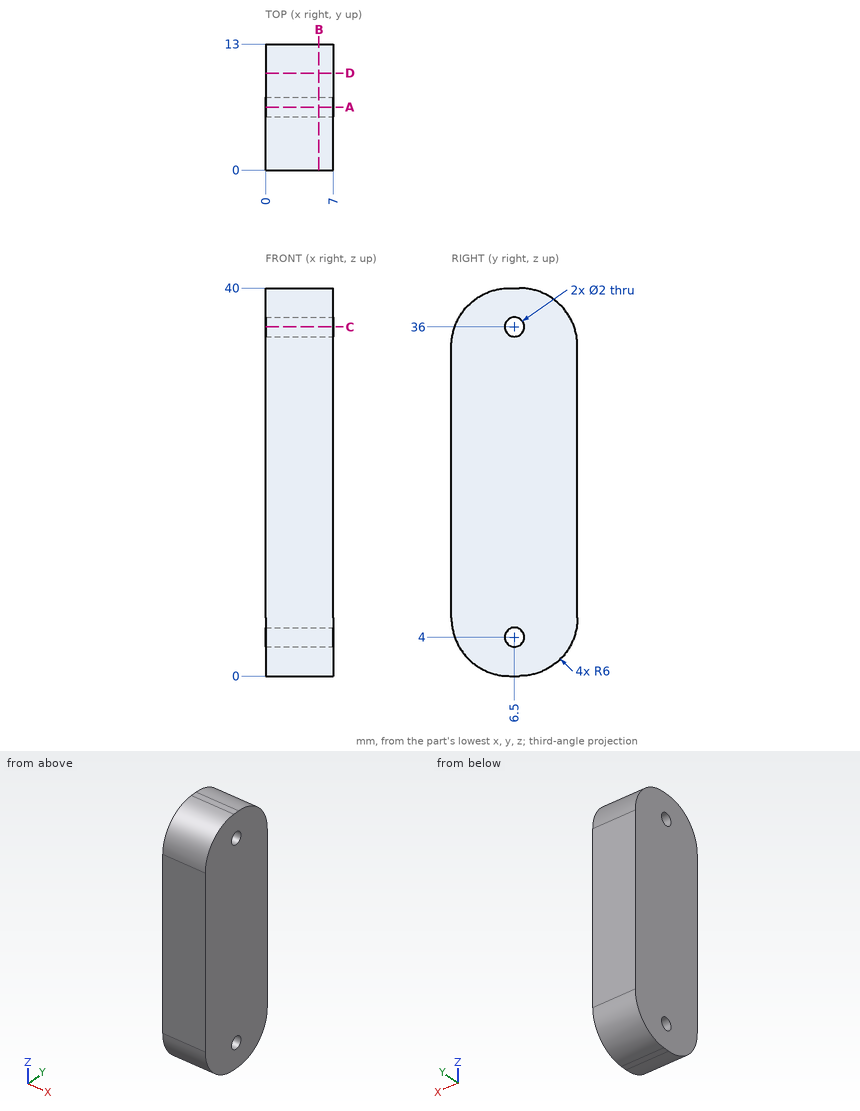
Design review of the part shown in the three views and the two pictorial views. Dimensions are in mm from the part's minimum x, y and z. Coordinates: 2 decimals unless noted, no trailing zeros. Order: outer loops, then holes, each group sorted by start corner. A loop starts at its lowest first (then second) coordinate and runs counter-clockwise, first axis right, second up. Notation, with made-up numbers: (11.5, 20.25) -> (64.5, 20.25) arc R31 cw to (64.5, 53.25) -> close; hole circle Ø4 at (-5, 64). An arc over 180 degrees is marked (long way). Use one line per item in the form item = value. Start each with the question number.
(1) Add section C-C on z = 36. State the section outline as (x, y) points.
(2) Add section A-A on y = 6.5. State the section outline as (x, z) points.
(3) Add section D-D on y = 10. State the section outline as (x, z) points, plus the area to 3 significant figures.
(4) Insertion check: pin 1 (2 mm diameter, centred on x = 1.5, z = 4.5, fed in from +Y); pin 2 (1.6 mm diameter, centred on y = 6.5, z = 36, fed in from -X); pin 3 (2 mm diameter, centred on y = 11.5, z = 8, fed in from -X). Each pin has a flat end and moves straight along its axis. Give the tip position at first contact, or say it passes through.
(5) Add section B-B on x = 5.5. State the section outline as (y, z) points, plus the area to 3 significant figures.
(6) For probe 1 along Z at (x, y) = (4.75, 6.5); probe 2 along Y at (x, z) = (3.25, 4.5); probe 3 along Z at (x, y) = (6.75, 7.75), list the stretches that pass through material, from the lowest coordinate up.
Answer block:
q1.outline = (0, 0.34) -> (7, 0.34) -> (7, 5.5) -> (0, 5.5) -> close; (0, 7.5) -> (7, 7.5) -> (7, 12.66) -> (0, 12.66) -> close
q2.outline = (0, 0) -> (7, 0) -> (7, 3) -> (0, 3) -> close; (0, 5) -> (7, 5) -> (7, 35) -> (0, 35) -> close; (0, 37) -> (7, 37) -> (7, 40) -> (0, 40) -> close
q3.outline = (0, 0.8) -> (7, 0.8) -> (7, 39.2) -> (0, 39.2) -> close
q3.area = 269 mm²
q4.pin_1 = 12.98
q4.pin_2 = through
q4.pin_3 = 0
q5.outline = (0, 6) arc R6 ccw to (6, 0) -> (7, 0) arc R6 ccw to (13, 6) -> (13, 34) arc R6 ccw to (7, 40) -> (6, 40) arc R6 ccw to (0, 34) -> close; hole circle Ø2 at (6.5, 4); hole circle Ø2 at (6.5, 36)
q5.area = 483 mm²
q6.probe_1 = 0 to 3, 5 to 35, 37 to 40
q6.probe_2 = 0.19 to 5.63, 7.37 to 12.81
q6.probe_3 = 0.05 to 39.95
